Check sheet for the modelled part. Datum: model origin and axes. Units: mm. Face numbers are marked on the shaded views. Give positions to 0.01 mm unless a question says otherwise; leave off trailing zeros. Write each loop counter-clockwise with the first axis right and the second up, starting at its lowest first coordinate (ties: lowest second). Pieces come first, ordered by that corner, then holes. Notation, with made-up numbers: (46, 83) -> (92, 83) arc R11 cw to (92, 96) -> close; hole circle Ø1 at (-4.75, 10). An arc over 180 degrees is marked (long way). Answer as a JSON object with one key per item and string values.
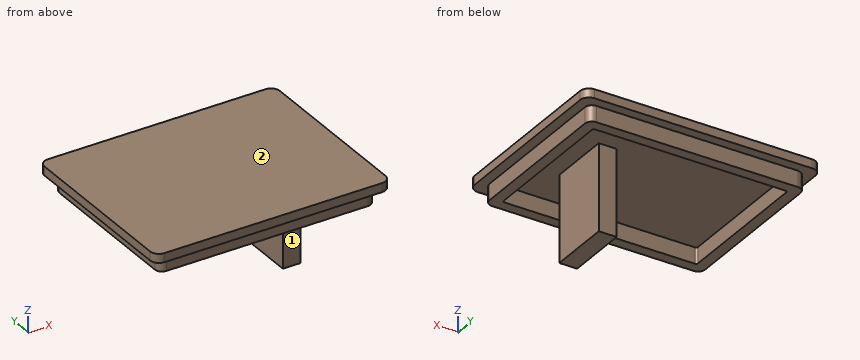
Autodesk Inventor part; units mm, degrees
ref_plane "YZ Plane" through (0, 0, 0) normal (1, 0, 0) x (0, 1, 0)
ref_plane "XZ Plane" through (0, 0, 0) normal (0, 1, 0) x (-1, 0, 0)
ref_plane "XY Plane" through (0, 0, 0) normal (0, 0, 1) x (1, 0, 0)
sketch "Sketch1" plane through (0, 0, 0) normal (0, 0, 1) x (1, 0, 0)
  line L0 (-66, 51.75) -> (66, 51.75)
  line L1 (66, 51.75) -> (66, -51.75)
  line L2 (66, -51.75) -> (-66, -51.75)
  line L3 (-66, -51.75) -> (-66, 51.75)
  line L4 (-60.5, 46.25) -> (60.5, 46.25)
  line L5 (60.5, 46.25) -> (60.5, -46.25)
  line L6 (60.5, -46.25) -> (-60.5, -46.25)
  line L7 (-60.5, -46.25) -> (-60.5, 46.25)
  line L8 (54.5, 40.25) -> (-54.5, 40.25)
  line L9 (-54.5, 40.25) -> (-54.5, -40.25)
  line L10 (-54.5, -40.25) -> (54.5, -40.25)
  line L11 (54.5, -40.25) -> (54.5, 40.25)
  line L12 (0, 46.25) -> (0, 40.25) construction
  line L13 (-60.5, 0) -> (-54.5, 0) construction
  line L14 (0, 51.75) -> (0, 46.25) construction
  line L15 (-60.5, 0) -> (-66, 0) construction
  line L16 (37, 17.5) -> (27, 17.5)
  line L17 (27, 17.5) -> (27, -17.5)
  line L18 (27, -17.5) -> (37, -17.5)
  line L19 (37, -17.5) -> (37, 17.5)
  line L20 (66, -46.75) -> (66, 46.75)
  line L21 (-61, -51.75) -> (61, -51.75)
  line L22 (-61, 46.75) -> (61, 46.75)
  line L23 (61, 46.75) -> (61, -46.75)
  point P0 (0, 0)
  point P1 (60.5, 0)
  point P2 (66, 0)
  point P3 (37, 0)
  point P4 (54.5, 0)
  dimension "d9" = 0.5
  dimension "d10" = 6
  dimension "d11" = 10
  dimension "d12" = 35
  dimension "d13" = 24
extrude "Extrusion1" add sketch "Sketch1" along normal blind 5 contours L0 L1 L2 L3 | L4 L5 L6 L7 | L11 L10 L9 L8 | L19 L18 L17 L16
extrude "Extrusion2" add sketch "Sketch1" against normal blind 9 contours L4 L5 L6 L7
extrude "Extrusion3" add sketch "Sketch1" against normal blind 48.5 contours L19 L18 L17 L16
fillet "Fillet1" radius 5 4 edges at (66, 51.75, 2.5) (-66, 51.75, 2.5) (66, -51.75, 2.5) (-66, -51.75, 2.5)
fillet "Fillet2" radius 4 4 edges at (-60.5, -46.25, -4.5) (60.5, -46.25, -4.5) (60.5, 46.25, -4.5) (-60.5, 46.25, -4.5)
fillet "Fillet3" radius 1 4 edges at (54.5, -40.25, -4.5) (-54.5, -40.25, -4.5) (54.5, 40.25, -4.5) (-54.5, 40.25, -4.5)
properties part number "kucisteGornji"
1. Mould release check, pull along X, two halves, no side actions. Record for the marked faces 1 and 2: released by +X, released by -X, zero draft, split by the parting line, or undercut.
Determined:
{"face 1": "undercut", "face 2": "zero draft"}
2. Sectioned sample at D-D, the plane y = -32. Enter the section's corners in (x, z).
Determined:
{"outline": "(-66, 0) -> (-60.5, 0) -> (-60.5, -9) -> (-54.5, -9) -> (-54.5, 0) -> (54.5, 0) -> (54.5, -9) -> (60.5, -9) -> (60.5, 0) -> (66, 0) -> (66, 5) -> (-66, 5) -> close"}
3. Sectioned sample at C-C, the plane y = 12. Enter the section's corners in (x, z), plus the area to 3 significant figures.
Determined:
{"outline": "(-66, 0) -> (-60.5, 0) -> (-60.5, -9) -> (-54.5, -9) -> (-54.5, 0) -> (27, 0) -> (27, -48.5) -> (37, -48.5) -> (37, 0) -> (54.5, 0) -> (54.5, -9) -> (60.5, -9) -> (60.5, 0) -> (66, 0) -> (66, 5) -> (-66, 5) -> close", "area": "1,250 mm^2"}
4. Sectioned sample at A-A, the plane z = -7. Enter the section's corners in (x, y).
Determined:
{"outline": "(-60.5, -42.25) arc R4 ccw to (-56.5, -46.25) -> (56.5, -46.25) arc R4 ccw to (60.5, -42.25) -> (60.5, 42.25) arc R4 ccw to (56.5, 46.25) -> (-56.5, 46.25) arc R4 ccw to (-60.5, 42.25) -> close; (27, -17.5) -> (37, -17.5) -> (37, 17.5) -> (27, 17.5) -> close; hole (-54.5, -39.25) arc R1 ccw to (-53.5, -40.25) -> (53.5, -40.25) arc R1 ccw to (54.5, -39.25) -> (54.5, 39.25) arc R1 ccw to (53.5, 40.25) -> (-53.5, 40.25) arc R1 ccw to (-54.5, 39.25) -> close"}
5. Go/stop test with flat-tipped pins: P1, Ø4.5, axis at y = 7, z = -2.5, coming from the +X side; P2, Ø4, axis at y = -13, z = -20.5, coming from the +X side; P3, Ø10, axis at y = 6.5, z = -6, coming from the -X side. Record where each tip stops, or that it passes through.
Determined:
{"P1": "x = 60.5", "P2": "x = 37", "P3": "x = -60.5"}
6. Sectioned sample at B-B, the plane x = -42.5. Enter the section's corners in (y, z), plus the area to 4 significant figures.
Determined:
{"outline": "(-51.75, 0) -> (-46.25, 0) -> (-46.25, -9) -> (-40.25, -9) -> (-40.25, 0) -> (40.25, 0) -> (40.25, -9) -> (46.25, -9) -> (46.25, 0) -> (51.75, 0) -> (51.75, 5) -> (-51.75, 5) -> close", "area": "625.5 mm^2"}
7. Scan lines: L1, parallel to X at y = -9.5, z = -8; L2, parallel to Y at x = -0.5, z = -6.5; L3, parallel to Z at x = -17, y = 4. Record each from-to range of solid material in increasing order. Write a range as [from, to].
Determined:
{"L1": "[-60.5, -54.5], [27, 37], [54.5, 60.5]", "L2": "[-46.25, -40.25], [40.25, 46.25]", "L3": "[0, 5]"}
